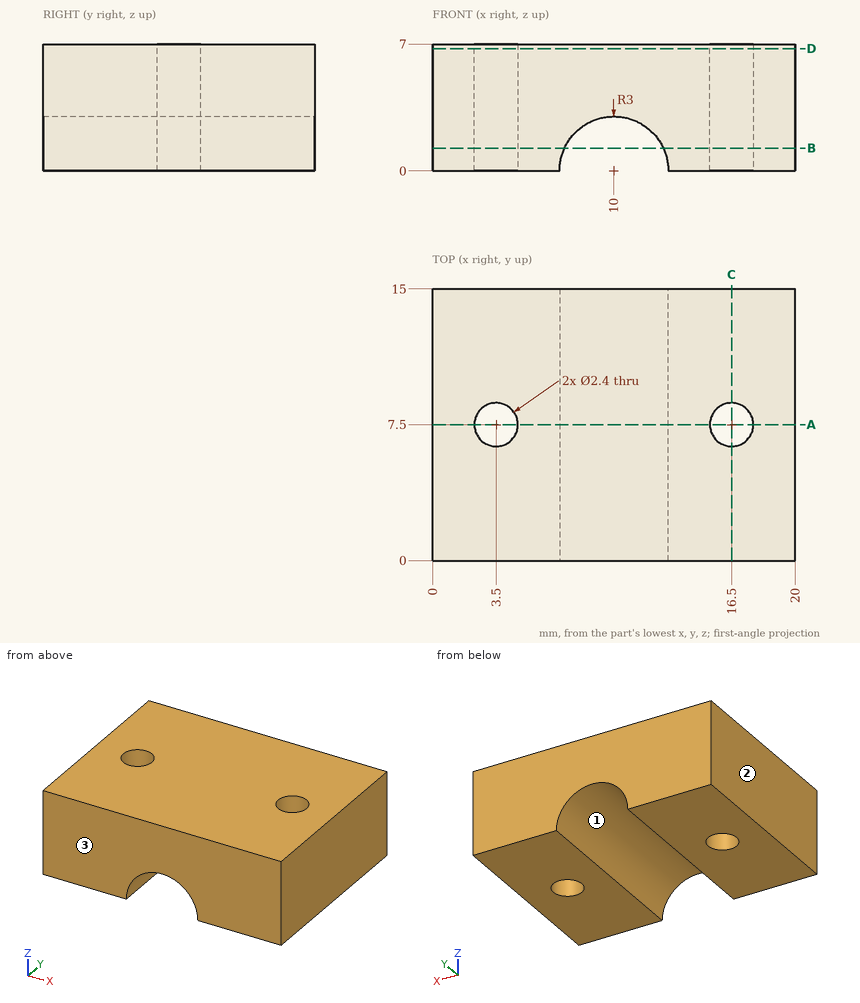
Could you check a few things on this drawing? It's one solid part, dimensions in mm from its lowest x, y, z. Coordinates: 2 decimals unless noted, no trailing zeros. Order: outer loops, then holes, each group sorted by start corner. A loop starts at its lowest first (then second) coordinate and runs counter-clockwise, first axis right, second up. Notation, with made-up numbers: M -26,30.5 L 5,30.5 A11 ccw 5,40.5 Z; hole C -10.5,55.5 d7. An arc over 180 degrees is marked long. Answer as a JSON object with one key per item and string values. Group by question number.
(1) Suppose I cut it at D-D, the plane z = 6.75. Please give me the cut outline in (x, y).
(2) I need wall thicknesses on probe 1 along Y at (x, z) = (16.5, 4.75); probe 2 along Y at (x, z) = (17, 1); probe 3 along Z at (x, y) = (10, 11). Which ranges of each line are inside material? Lowest first, please.
(3) Suppose I cut it at B-B, the plane z = 1.25. Please give me the cut outline in (x, y).
(4) For pin 1 (1.4 mm diameter, centred on x = 3.5, y = 7.5, fed in from -Z), with a flat end and sliding along its axis, tell me the tip position at first contact or that it passes through.
(5) Suppose I cut it at A-A, the plane y = 7.5. Please give me the cut outline in (x, z).
(6) If we mould it in two halves opening along X, with no side actions, what happens to the marked faces 1, 2 and 3? For each: released by +X, released by -X, zero draft, split by the parting line, or undercut.
(7) Suppose I cut it at C-C, the plane x = 16.5. Please give me the cut outline in (y, z), then the cut area to 3 significant figures.
Values found:
{
 "1": {"outline": "M 0,0 L 20,0 L 20,15 L 0,15 Z; hole C 3.5,7.5 d2.4; hole C 16.5,7.5 d2.4"},
 "2": {"probe 1": "y = 0 to 6.3, 8.7 to 15", "probe 2": "y = 0 to 6.41, 8.59 to 15", "probe 3": "z = 3 to 7"},
 "3": {"outline": "M 0,0 L 7.27,0 L 7.27,15 L 0,15 Z; M 12.73,0 L 20,0 L 20,15 L 12.73,15 Z; hole C 3.5,7.5 d2.4; hole C 16.5,7.5 d2.4"},
 "4": {"pin 1": "passes through"},
 "5": {"outline": "M 0,0 L 2.3,0 L 2.3,7 L 0,7 Z; M 4.7,0 L 7,0 A3 cw 13,0 L 15.3,0 L 15.3,7 L 4.7,7 Z; M 17.7,0 L 20,0 L 20,7 L 17.7,7 Z"},
 "6": {"face 1": "undercut", "face 2": "released by -X", "face 3": "zero draft"},
 "7": {"outline": "M 0,0 L 6.3,0 L 6.3,7 L 0,7 Z; M 8.7,0 L 15,0 L 15,7 L 8.7,7 Z", "area": "88.2 mm^2"}
}
